Geometry check sheet. Reference: drawing and pictorial views, mm from the part's lowest x, y, z. A direction names the side the tool comes from. Coordinates: 2 decimals unless noted, no trailing zeros. Loops run counter-clockwise (first coordinate to the right, second up) from the corner with the lowest first, then second, coordinate; pieces in that order, holes last. Notation, with made-up numbers: (76, 45) -> (88, 45) arc R15 cw to (88, 65) -> close; hole circle Ø7 at (67.5, 4). An arc over 180 degrees is marked (long way). Answer as a JSON object with one key per item and string values. Group by question number.
Q1. Set-up check for the marked faces 1 and 2: record each of +Z, -Z, +X, -X, +Y, -Y from which the full face is reachable in a straight line by a thin tool's end or side.
Q2. Scan lines: L1, parallel to X at y = 5.5, z = 5; L2, parallel to Z at x = 9.25, y = 7.25. Record each from-to range of solid material in increasing order.
Q3. Release check for a two-part mould opening along Y. For the marked faces 3, 4 and 5 record: released by +Y, released by -Y, zero draft, split by the parting line, or undercut.
Q4. Gauge pin test, flat ends, axial feed: pin 1 Ø2 at (y, z) = (6, 9) entering from -X; pin 2 Ø2 at (x, z) = (3.5, 7.5) entering from +Y; pin 3 Ø4 at (y, z) = (4.5, 6.5) entering from +X; pin 4 Ø5.5 at (x, y) = (7.5, 5.5) entering from -Z. Record the tip position at first contact, or that the pin passes through.
Q5. Cross-section at C-C on z = 9.75. Record the boundary of the cut face in (x, y).
Q6. Cross-section at A-A on y = 5.5. Record the boundary of the cut face in (x, z).
Q7. Cross-section at D-D on x = 1.75. Record the boundary of the cut face in (y, z), and give its area (3 significant figures).
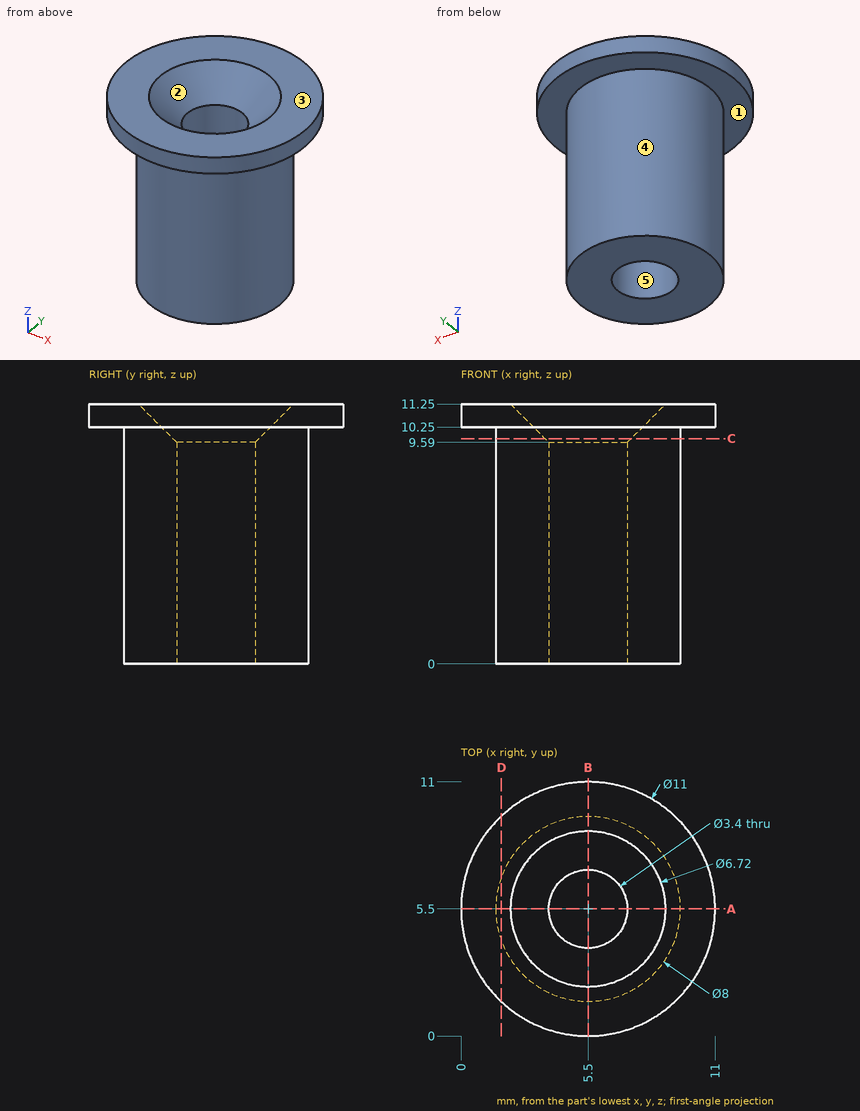
Computed values:
{
 "1": {"face 1": "-Z", "face 2": "+Z"},
 "2": {"L1": "x = 1.5 to 3.8, 7.2 to 9.5", "L2": "z = 10.25 to 11.25"},
 "3": {"face 3": "zero draft", "face 4": "split by the parting line", "face 5": "undercut"},
 "4": {"pin 1": "stops at x = 1.5", "pin 2": "stops at y = 9.37", "pin 3": "stops at x = 9.5", "pin 4": "stops at z = 0"},
 "5": {"outline": "circle Ø8 at (5.5, 5.5); hole circle Ø3.72 at (5.5, 5.5)"},
 "6": {"outline": "(0, 10.25) -> (1.5, 10.25) -> (1.5, 0) -> (3.8, 0) -> (3.8, 9.59) -> (2.14, 11.25) -> (0, 11.25) -> close; (7.2, 0) -> (9.5, 0) -> (9.5, 10.25) -> (11, 10.25) -> (11, 11.25) -> (8.86, 11.25) -> (7.2, 9.59) -> close"},
 "7": {"outline": "(1.48, 10.25) -> (4.11, 10.25) -> (4.11, 0) -> (6.89, 0) -> (6.89, 10.25) -> (9.52, 10.25) -> (9.52, 11.25) -> (1.48, 11.25) -> close", "area": "36.6 mm²"}
}
